Design review of the part built by this model. Coordinates are the model's own, in mm. Face numbers are marked on the shaded views. A direction names the side the tool comes from. Round coordinates to 2 decimals unless told otherwise and drop trailing zeros. Loops run counter-clockwise (first coordinate to the right, second up) from the corner with the lowest first, then second, coordinate; pieces in that order, holes last. Notation, with made-up numbers: (66, -39) - (81, -39) arc R21 cw to (81, -27) - close; hole circle Ø6 at (-19, 65.5). An arc over 180 degrees is marked (long way). Return JSON: item names as keys, results as strings. Group by question number.
(1) We need section C-C, the plane y = -5.25. Write out the cut boundary in (x, z), and give its area (3 significant figures).
(2) We need section B-B, the plane z = 1. Write out the cut boundary in (x, y), and give its area (4 significant figures).
(3) Wall thickness on L1, parallel to X at y = -1.75, z = 3.25; L2, parallel to X at y = -0.25, z = 2.75; L3, parallel to Z at x = -32, y = -1.25: over which ranges is each line inside the solid? List them lowest first. Write a range as [from, to].
(4) We need section D-D, the plane y = -2. Write out the cut boundary in (x, z).
(5) Clearance check with flat-ended pins moving along their axes: pin 1 (1 mm diameter, centred on x = 3.5, y = -3, fed in from +Z); pin 2 (2 mm diameter, centred on y = -4.5, z = 2, fed in from +X); pin 3 (1.5 mm diameter, centred on x = 16.5, z = 1, fed in from -Y); pin 4 (4 mm diameter, centred on x = -6, y = -2.5, fed in from -Z). State where each tip first meets the part, or that it passes through.
(6) We need section A-A, the plane x = 19.5. Write out the cut boundary in (y, z).
(7) The part is to be moulded in two halves that separate along Z. For the marked faces 1, 2 and 3, say which applies: pulls with the +Z half, pulls with the -Z half, needs draft (parallel to the pull), parting line crosses it, or undercut.
(8) For the marked faces 4, 5 and 6, list the 3-axis set-ups (+Z, -Z, +X, -X, +Y, -Y) from which the entire face can be reached by the end or side of a thin tool; tool diameter is ignored.
from build123d import *

# Parameters (mm, degrees)
F0_W     = 0.75
F0_H     = 3
F0_W_2   = 11.2
F0_H_2   = 1.5
F1_DEPTH = 7
F0_W_3   = 40
F2_DEPTH = 3
F0_W_4   = 9.8
F0_H_3   = 1.969696
F3_DEPTH = 7


with BuildPart() as f1:
    # F0 (on Front) → F1 (new body)
    with BuildSketch(Plane.XZ):
        with BuildLine():
            Line((-40.368542, 4.5), (-40.368542, 6))
            ThreePointArc((-40.368542, 6), (-41.822706, 4.802776), (-42.368542, 3))
            Line((-42.368542, 3), (-41.618542, 3))
            ThreePointArc((-41.618542, 3), (-41.166325, 3.893986), (-40.368542, 4.5))
        make_face()
        with Locations((-41.993542, 1.5)):
            Rectangle(F0_W, F0_H)
        with BuildLine():
            ThreePointArc((-42.368542, 0), (-41.822706, -1.802776), (-40.368542, -3))
            Line((-40.368542, -3), (-40.368542, -1.5))
            ThreePointArc((-40.368542, -1.5), (-41.162473, -0.890775), (-41.618542, 0))
            Line((-41.618542, 0), (-42.368542, 0))
        make_face()
        with Locations((-34.768542, -2.25)):
            Rectangle(F0_W_2, F0_H_2)
        with BuildLine():
            ThreePointArc((-29.168542, -3), (-27.815266, -1.778994), (-27.418542, 0))
            Line((-27.418542, 0), (-27.418542, 3))
            ThreePointArc((-27.418542, 3), (-27.815266, 4.778994), (-29.168542, 6))
            Line((-29.168542, 6), (-29.168542, 4.5))
            Line((-29.168542, 4.5), (-29.168542, -1.5))
            Line((-29.168542, -1.5), (-29.168542, -3))
        make_face()
        with Locations((-34.768542, 5.25)):
            Rectangle(F0_W_2, F0_H_2)
        with BuildLine():
            ThreePointArc((-41.618542, 0), (-41.162473, -0.890775), (-40.368542, -1.5))
            Line((-40.368542, -1.5), (-40.368542, 4.5))
            ThreePointArc((-40.368542, 4.5), (-41.166325, 3.893986), (-41.618542, 3))
            Line((-41.618542, 3), (-41.618542, 0))
        make_face()
    extrude(amount=F1_DEPTH)

    # F0 (on Front) → F2 (join)
    with BuildSketch(Plane.XZ):
        with Locations((-7.418542, 1.5)):
            Rectangle(F0_W_3, F0_H)
    extrude(amount=F2_DEPTH)

    # F0 (on Front) → F3 (join)
    with BuildSketch(Plane.XZ):
        with BuildLine():
            Line((12.581458, 3), (12.581458, 0))
            ThreePointArc((12.581458, 0), (13.065893, -1.47902), (14.331458, -2.384848))
            Line((14.331458, -2.384848), (14.331458, -0.415152))
            Line((14.331458, -0.415152), (14.331458, 3.884848))
            Line((14.331458, 3.884848), (14.331458, 5.384848))
            ThreePointArc((14.331458, 5.384848), (13.065893, 4.47902), (12.581458, 3))
        make_face()
        with Locations((19.231458, -1.4)):
            Rectangle(F0_W_4, F0_H_3)
        with BuildLine():
            Line((24.131458, -0.415152), (24.131458, -2.384848))
            ThreePointArc((24.131458, -2.384848), (25.687695, -1.6589), (26.131458, 0))
            Line((26.131458, 0), (25.381458, 0))
            Line((25.381458, 0), (25.381458, 3))
            Line((25.381458, 3), (26.131458, 3))
            ThreePointArc((26.131458, 3), (25.687695, 4.6589), (24.131458, 5.384848))
            Line((24.131458, 5.384848), (24.131458, 3.884848))
            Line((24.131458, 3.884848), (24.131458, -0.415152))
        make_face()
        with Locations((25.756458, 1.5)):
            Rectangle(F0_W, F0_H)
        with Locations((19.231458, 4.634848)):
            Rectangle(F0_W_4, F0_H_2)
    extrude(amount=F3_DEPTH)


solid = f1.part
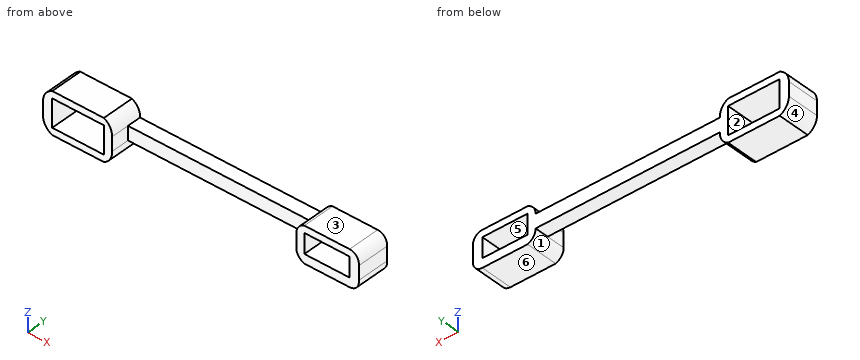
Solutions:
{
 "1": {"outline": "(-42.37, 0) arc R3.25 ccw to (-40.37, -3) - (-29.17, -3) arc R3 ccw to (-27.42, 0) - (-27.42, 3) arc R3 ccw to (-29.17, 6) - (-40.37, 6) arc R3.25 ccw to (-42.37, 3) - close; (12.58, 0) arc R2.5 ccw to (14.33, -2.38) - (24.13, -2.38) arc R2.03 ccw to (26.13, 0) - (26.13, 3) arc R2.03 ccw to (24.13, 5.38) - (14.33, 5.38) arc R2.5 ccw to (12.58, 3) - close; hole (-40.37, -1.5) - (-29.17, -1.5) - (-29.17, 4.5) - (-40.37, 4.5) - close; hole (14.33, -0.42) - (24.13, -0.42) - (24.13, 3.88) - (14.33, 3.88) - close", "area": "121 mm^2"},
 "2": {"outline": "(-42.37, -7) - (-40.37, -7) - (-40.37, 0) - (-42.37, 0) - close; (-29.17, -7) - (-27.42, -7) - (-27.42, -3) - (12.58, -3) - (12.58, -7) - (14.33, -7) - (14.33, 0) - (-29.17, 0) - close; (24.13, -7) - (26.13, -7) - (26.13, 0) - (24.13, 0) - close", "area": "172.5 mm^2"},
 "3": {"L1": "[-42.36, -40.37], [-29.17, -27.41], [12.59, 14.33], [24.13, 26.16]", "L2": "[-42.37, -40.37], [-29.17, 14.33], [24.13, 26.13]", "L3": "[-3, -1.5], [4.5, 6]"},
 "4": {"outline": "(-42.37, 0) arc R3.25 ccw to (-40.37, -3) - (-29.17, -3) arc R3 ccw to (-27.42, 0) - (12.58, 0) arc R2.5 ccw to (14.33, -2.38) - (24.13, -2.38) arc R2.03 ccw to (26.13, 0) - (26.13, 3) arc R2.03 ccw to (24.13, 5.38) - (14.33, 5.38) arc R2.5 ccw to (12.58, 3) - (-27.42, 3) arc R3 ccw to (-29.17, 6) - (-40.37, 6) arc R3.25 ccw to (-42.37, 3) - close; hole (-40.37, -1.5) - (-29.17, -1.5) - (-29.17, 4.5) - (-40.37, 4.5) - close; hole (14.33, -0.42) - (24.13, -0.42) - (24.13, 3.88) - (14.33, 3.88) - close"},
 "5": {"pin 1": "z = 3", "pin 2": "x = 26.13", "pin 3": "through", "pin 4": "z = 0"},
 "6": {"outline": "(-7, -2.38) - (0, -2.38) - (0, -0.42) - (-7, -0.42) - close; (-7, 3.88) - (0, 3.88) - (0, 5.38) - (-7, 5.38) - close"},
 "7": {"face 1": "pulls with the -Z half", "face 2": "undercut", "face 3": "pulls with the +Z half"},
 "8": {"face 4": "-Z, -X, +Y, -Y", "face 5": "+Y, -Y", "face 6": "-Z, +X, +Y, -Y"}
}
